For this review, take the finished solid that the model builds, in its own axes (mm). A direction names the side the tool comes from. Round coordinates to 2 decimals unless told otherwise and drop trailing zeros. Write each loop counter-clockwise with the first axis right and the second up, starting at its lowest first coordinate (ties: lowest second). Pieces come first, ordered by that corner, then holes. Notation, with made-up numbers: (79.25, -14) -> (128.25, -14) arc R34 ccw to (128.25, 21) -> close; hole circle Ø6 at (7.25, 62.25). An arc over 180 degrees is marked (long way). Write each question's results on one line, items separated by ' | '. Start each with the question number.
Item 1: Add section C-C (y = -53.5). State the section outline as (x, z) points.
Item 2: Add section A-A (y = -65). State the section outline as (x, z) points, plus the area to 3 significant figures.
Item 3: Add section D-D (x = -32). State the section outline as (y, z) points, plus the area to 3 significant figures.
Item 4: Tool access review of faces 1 (the flat face through (-33.946, -66, -50)), 2 (the flat face through (-37.346, -66, -54)), 3 (the flat face through (-27.746, -54, -48)): name each direction out of +Z, -Z, +X, -X, +Y, -Y from which nothing blocks a thin tool from reaching the whole face with its end or side.
Item 5: To check wall thickness, follow line 1 along Y through (x, z) = (-35.7, -52); line 2 along X through (y, z) = (-53.5, -48.5); line 3 along Y through (x, z) = (-34.8, -52). State the ranges of each line that lie inside material, in increasing order.
Item 6: The part is to be moulded in two halves that separate along Y. For faces 4 (the cylindrical face through (-35.623, -66.088, -53.617)), 5 (the cylindrical face through (-35.67, -69.046, -53.684)), 6 (the flat face through (-31.1, -57.9, -48.6)), say which applies: +Y half, -Y half, draft (parallel to the pull), parting line (faces both ways), or undercut.
Item 7: Clearance check with flat-ended pins moving along their axes: pin 1 (5 mm diameter, centred on y = -55.5, z = -52, fed in from -X); pin 2 (1 mm diameter, centred on x = -35, z = -48, fed in from +Y); pin 3 (3 mm diameter, centred on y = -52.74, z = -46.45, fed in from -X); pin 4 (1 mm diameter, centred on y = -53, z = -51, fed in from -X). State where each tip first meets the part, or that it passes through.
from build123d import *

# Parameters (mm, degrees)
BOSS_EXTRUDE1_DEPTH = 13
SKETCH2_W           = 9.6
SKETCH2_H           = 12.263448081
CUT_EXTRUDE1_DEPTH  = 94.999820378
DRAFT1_ANGLE        = 20
CUT_EXTRUDE2_DEPTH  = 94.999820378
HOLE1_D             = 3.5
HOLE2_D             = 3.5
FILLET1_R           = 0.6
FILLET2_R           = 5


with BuildPart() as part:
    # Sketch1 → Boss-Extrude1 (new body)
    with BuildSketch(Plane(origin=(-37.346370889, 0, 0), x_dir=(0, -1, 0), z_dir=(-1, 0, 0))):
        with BuildLine():
            Line((51.136566376, -50.11421745), (63.813413447, -55.66421745))
            ThreePointArc((63.813413447, -55.66421745), (69.081847366, -53.604216469), (67.021846385, -48.33578255))
            Line((67.021846385, -48.33578255), (54.344999314, -42.78578255))
            ThreePointArc((54.344999314, -42.78578255), (49.076565395, -44.845783531), (51.136566376, -50.11421745))
        make_face()
    extrude(amount=-BOSS_EXTRUDE1_DEPTH)

    # Sketch2 → Cut-Extrude1 (cut, through all)
    with BuildSketch(Plane(origin=(0, 6.977867205, -15.938262243), x_dir=(1, 0, 0), z_dir=(0, -0.4010541172489907, 0.9160543624903671))):
        with Locations((-32.546370889, -68.673916916)):
            Rectangle(SKETCH2_W, SKETCH2_H)
    extrude(amount=-CUT_EXTRUDE1_DEPTH, mode=Mode.SUBTRACT)

    # Draft1
    draft1_faces = [part.faces().sort_by_distance(p)[0] for p in [
        (-32.546370889, -59.943950062, -49.603589992),
    ]]
    draft(draft1_faces, Plane(origin=(-37.346370889, -52.740782845, -46.45), x_dir=(0, -1, 0), z_dir=(-1, 0, 0)), DRAFT1_ANGLE)

    # Sketch3 → Cut-Extrude2 (cut, through all)
    with BuildSketch(Plane(origin=(0, 6.977867205, -15.938262243), x_dir=(1, 0, 0), z_dir=(0, -0.4010541172489907, 0.9160543624903671))):
        Polygon((-18.270337706, -85.869129535), (-18.270337706, -71.075309896), (-33.946370889, -76.780919366), (-33.946370889, -85.869129535), align=None)
    extrude(amount=-CUT_EXTRUDE2_DEPTH, mode=Mode.SUBTRACT)

    # Hole1 (through all)
    with Locations(Plane.ZY.offset(37.346370889)):
        with Locations((-52, -65.417629916)):
            Hole(HOLE1_D / 2)

    # Hole2 (through all)
    with Locations(Plane(origin=(-24.346370889, 0, 0), x_dir=(0, 0, -1), z_dir=(1, 0, 0))):
        with Locations((46.45, -52.740782845)):
            Hole(HOLE2_D / 2)

    # Fillet1
    fillet1_edges = [part.edges().sort_by_distance(p)[0] for p in [
        (-27.746370889, -56.743151462, -48.202261087),
        (-33.946370889, -61.753412466, -50.395783531),
    ]]
    fillet(fillet1_edges, radius=FILLET1_R)

    # Fillet2
    fillet2_edges = [part.edges().sort_by_distance(p)[0] for p in [
        (-37.346370889, -59.943950062, -49.603589992),
        (-24.346370889, -58.552613866, -48.994454625),
    ]]
    fillet(fillet2_edges, radius=FILLET2_R)


solid = part.part
Responses:
1) outline: (-27.75, -51.15) -> (-24.35, -51.15) -> (-24.35, -48.03) -> (-27.75, -48.03) -> close; (-27.75, -44.87) -> (-24.35, -44.87) -> (-24.35, -42.52) -> (-27.75, -42.52) -> close
2) outline: (-37.35, -55.98) -> (-33.95, -55.98) -> (-33.95, -53.7) -> (-37.35, -53.7) -> close; (-37.35, -50.3) -> (-33.95, -50.3) -> (-33.95, -47.45) -> (-37.35, -47.45) -> close | area: 17.4 mm^2
3) outline: (-62.71, -46.45) -> (-59.5, -53.78) -> (-56.56, -52.49) -> (-59.77, -45.16) -> close | area: 25.7 mm^2
4) face 1: -Z, +X, -Y | face 2: +Z, -Z, -X, +Y, -Y | face 3: +Z, -X, +Y
5) line 1: y = -69.42 to -67.17, -63.67 to -58.67 | line 2: x = -27.75 to -24.35 | line 3: y = -69.42 to -67.17, -63.67 to -57.96
6) face 4: undercut | face 5: parting line | face 6: +Y half
7) pin 1: stops at x = -35.19 | pin 2: stops at y = -59.46 | pin 3: passes through | pin 4: stops at x = -27.75
